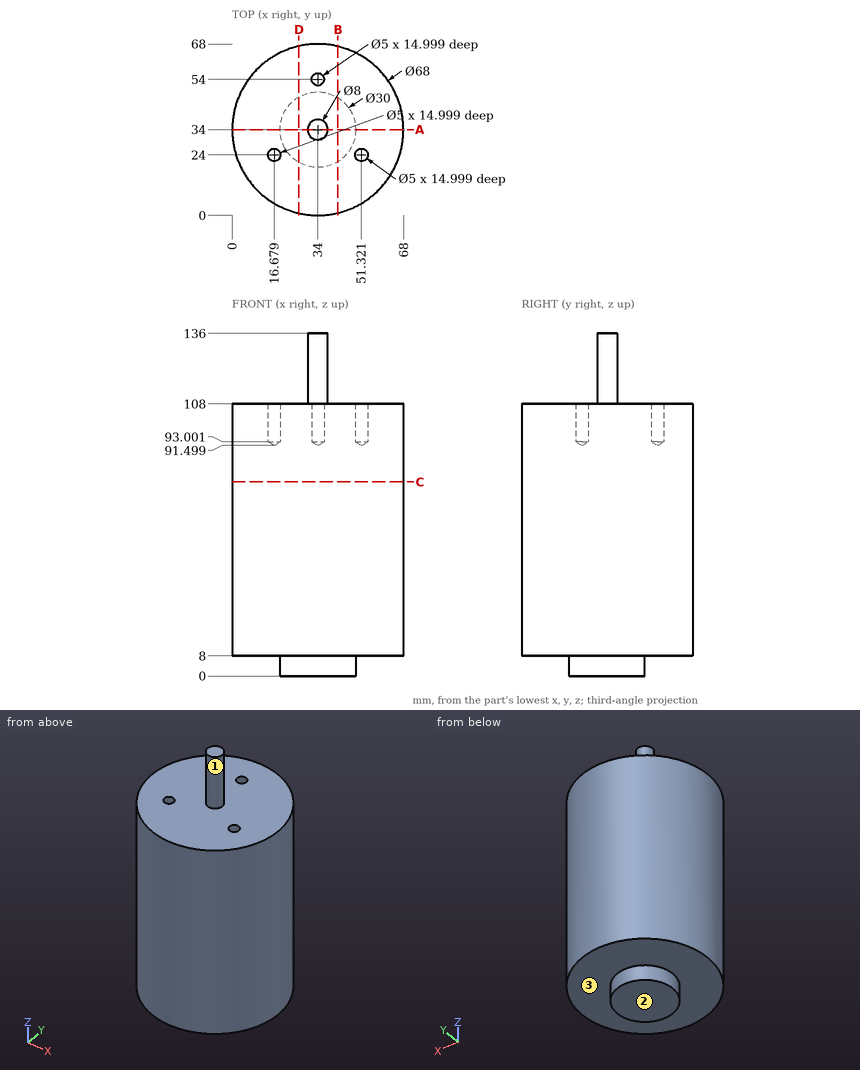
Geometry check sheet. Reference: drawing and pictorial views, mm from the part's lowest x, y, z. A direction names the side the tool comes from. Round coordinates to 2 decimals unless told otherwise and drop trailing zeros. Write each loop counter-clockwise with the first axis right and the second up, starting at its lowest first coordinate (ties: lowest second). Pieces come first, ordered by that corner, then holes.
(1) Section check D-D (x = 26.5). Enter the section's corners in (y, z).
Returned:
outline: (0.84, 8) - (21.01, 8) - (21.01, 0) - (46.99, 0) - (46.99, 8) - (67.16, 8) - (67.16, 108) - (0.84, 108) - close
(2) Material ranges on line 1 (X direction, y = 24, z = 103.75) (1 decimal); line 2 (Z direction, x = 47.5, y = 51.5); line 3 (Z direction, x = 43.5, y = 30), recorded low to high.
Returned:
line 1: x = 1.5 to 14.2, 19.2 to 48.8, 53.8 to 66.5
line 2: z = 8 to 108
line 3: z = 0 to 108
(3) Access from +Z, -Z, +X, -X, +Y, -Y to the whole of each face (thin tool, end or side, straight path). Record for the marked faces 1, 2 and 3.
Returned:
face 1: +Z
face 2: -Z, +X, -X, +Y, -Y
face 3: -Z
(4) Section check A-A (y = 34). Enter the section's corners in (x, z), plus the area to 3 significant figures.
Returned:
outline: (0, 8) - (19, 8) - (19, 0) - (49, 0) - (49, 8) - (68, 8) - (68, 108) - (38, 108) - (38, 136) - (30, 136) - (30, 108) - (0, 108) - close
area: 7,260 mm2
(5) Section check C-C (z = 77). Enter the section's corners in (x, y), plus the area to 3 significant figures.
Returned:
outline: circle Ø68 at (34, 34)
area: 3,630 mm2
(6) Depth check by flat-ended pin: pin 1 Ø4 at (x, y) = (16.68, 24) entering from +Z; pin 2 Ø4 at (x, y) = (34, 54) entering from -Z; pin 3 Ø20.5 at (x, y) = (28, 25) entering from -Z; pin 4 Ø3 at (x, y) = (9, 8.5) entering from +Z. Enter the tip coordinate at first touch or a pass-through.
Returned:
pin 1: stops at z = 92.7
pin 2: stops at z = 8
pin 3: stops at z = 0
pin 4: passes through
(7) Section check B-B (x = 42). Enter the section's corners in (y, z) (1 decimal), plus the area to 3 significant figures.
Returned:
outline: (1, 8) - (21.3, 8) - (21.3, 0) - (46.7, 0) - (46.7, 8) - (67, 8) - (67, 108) - (1, 108) - close
area: 6,810 mm2
